from build123d import *

# Parameters (mm, degrees)
F0_R       = 5
F1_DEPTH   = 10
F2_R       = 7.5
F3_DEPTH   = 2
F4_C1_SIZE = 1
F4_C2_SIZE = 1
F4_C3_SIZE = 1
F4_C4_SIZE = 1
F4_C5_SIZE = 1
F4_C6_SIZE = 1
F4_C7_SIZE = 0.9999
F4_C8_SIZE = 1


# Not quite as in the source:
# - a fillet or chamfer is up to 0.001 mm smaller than in the source, because OpenCascade refuses the exact size


with BuildPart() as f1:
    # F0 (on Front) → F1 (new body)
    with BuildSketch(Plane.XZ):
        with BuildLine():
            ThreePointArc((3.1540486056, 9.4895720343), (1.5765683293, 9.7419684548), (0, 10))
            ThreePointArc((0, 10), (-10, 0), (0, -10))
            ThreePointArc((0, -10), (1.5765683293, -9.7419684548), (3.1540486056, -9.4895720343))
            ThreePointArc((3.1540486056, -9.4895720343), (8.1098855126, -5.8506202211), (10, 0))
            ThreePointArc((10, 0), (8.1098855126, 5.8506202211), (3.1540486056, 9.4895720343))
        make_face()
        Circle(F0_R, mode=Mode.SUBTRACT)
        with BuildLine():
            ThreePointArc((3.1540486056, 9.4895720343), (1.5975418081, 9.8715682731), (0, 10))
            ThreePointArc((0, 10), (1.5765683293, 9.7419684548), (3.1540486056, 9.4895720343))
        make_face()
        with BuildLine():
            ThreePointArc((3.1540486056, -9.4895720343), (1.5765683293, -9.7419684548), (0, -10))
            ThreePointArc((0, -10), (1.5975418081, -9.8715682731), (3.1540486056, -9.4895720343))
        make_face()
        with BuildLine():
            ThreePointArc((142.8459513944, 9.4895720343), (73, 4), (3.1540486056, 9.4895720343))
            ThreePointArc((3.1540486056, 9.4895720343), (8.1098855126, 5.8506202211), (10, 0))
            ThreePointArc((10, 0), (8.1098855126, -5.8506202211), (3.1540486056, -9.4895720343))
            ThreePointArc((3.1540486056, -9.4895720343), (73, -4), (142.8459513944, -9.4895720343))
            ThreePointArc((142.8459513944, -9.4895720343), (136, 0), (142.8459513944, 9.4895720343))
        make_face()
        with BuildLine():
            ThreePointArc((146, 10), (144.4234316707, 9.7419684548), (142.8459513944, 9.4895720343))
            ThreePointArc((142.8459513944, 9.4895720343), (136, 0), (142.8459513944, -9.4895720343))
            ThreePointArc((142.8459513944, -9.4895720343), (144.4234316707, -9.7419684548), (146, -10))
            ThreePointArc((146, -10), (153.0710678119, -7.0710678119), (156, 0))
            ThreePointArc((156, 0), (153.0710678119, 7.0710678119), (146, 10))
        make_face()
        with Locations((146, 0)):
            Circle(F0_R, mode=Mode.SUBTRACT)
        with BuildLine():
            ThreePointArc((146, 10), (144.4024581919, 9.8715682731), (142.8459513944, 9.4895720343))
            ThreePointArc((142.8459513944, 9.4895720343), (144.4234316707, 9.7419684548), (146, 10))
        make_face()
        with BuildLine():
            ThreePointArc((146, -10), (144.4234316707, -9.7419684548), (142.8459513944, -9.4895720343))
            ThreePointArc((142.8459513944, -9.4895720343), (144.4024581919, -9.8715682731), (146, -10))
        make_face()
    extrude(amount=F1_DEPTH)

    # F2 (on face) → F3 (cut)
    with BuildSketch(Plane.XZ.offset(10)):
        Circle(F2_R)
        with Locations((146, 0)):
            Circle(F2_R)
    extrude(amount=-F3_DEPTH, mode=Mode.SUBTRACT)

    # F4: chamfer of 1 on 8 edges, made by hand

    # F4_c1
    f4_c1_edges = [f1.edges().sort_by_distance(p)[0] for p in [
        (73, 0, -4),
    ]]
    chamfer(f4_c1_edges, length=F4_C1_SIZE)

    # F4_c2
    f4_c2_edges = [f1.edges().sort_by_distance(p)[0] for p in [
        (73, 0, 3.9999999999),
    ]]
    chamfer(f4_c2_edges, length=F4_C2_SIZE)

    # F4_c3
    f4_c3_edges = [f1.edges().sort_by_distance(p)[0] for p in [
        (-5, 0, 0),
    ]]
    chamfer(f4_c3_edges, length=F4_C3_SIZE)

    # F4_c4
    f4_c4_edges = [f1.edges().sort_by_distance(p)[0] for p in [
        (141, 0, 0),
    ]]
    chamfer(f4_c4_edges, length=F4_C4_SIZE)

    # F4_c5
    f4_c5_edges = [f1.edges().sort_by_distance(p)[0] for p in [
        (-5, -8, 0),
    ]]
    chamfer(f4_c5_edges, length=F4_C5_SIZE)

    # F4_c6
    f4_c6_edges = [f1.edges().sort_by_distance(p)[0] for p in [
        (141, -8, 0),
    ]]
    chamfer(f4_c6_edges, length=F4_C6_SIZE)

    # F4_c7 (size 1 in the source; OpenCascade refuses exactly that, so slightly less here)
    f4_c7_edges = [f1.edges().sort_by_distance(p)[0] for p in [
        (-10, 0, 0),
    ]]
    chamfer(f4_c7_edges, length=F4_C7_SIZE)

    # F4_c8
    f4_c8_edges = [f1.edges().sort_by_distance(p)[0] for p in [
        (156, 0, 0),
    ]]
    chamfer(f4_c8_edges, length=F4_C8_SIZE)


solid = f1.part
Work out the finished part from the listing and answer in its coordinate system (mm). A direction names the side the tool comes from. Round coordinates to 2 decimals unless told otherwise and drop trailing zeros. Write each loop counter-clockwise with the first axis right and the second up, starting at its lowest first coordinate (ties: lowest second). Pieces come first, ordered by that corner, then holes. Notation, with made-up numbers: M 64,9 L 77,9 A16 ccw 77,25 Z; hole C 16.25,56.5 d2. An arc over 180 degrees is marked long. Use a Markdown table: item, result.
1) Determine the mould class of faces 3 (the face through (74, -0.8, 3.8)), 4 (the face through (72, -10, 0)) for opening direction X: pulls with the +X half, pulls with the -X half, needs draft (parallel to the pull), parting line crosses it, or undercut.
Taken from the geometry:
| item | result |
|---|---|
| face 3 | undercut |
| face 4 | needs draft |
2) The part is cut by section A-A on y = -3.75. Give the vertices of the cut face in (x, z), plus the area to 3 significant figures.
Taken from the geometry:
| item | result |
|---|---|
| outline | M 3.15,-9.49 A447.08 cw 142.85,-9.49 A10 ccw long 142.85,9.49 A447.08 cw 3.15,9.49 A10 ccw long Z; hole C 0,0 d10; hole C 146,0 d10 |
| area | 1,910 mm2 |
3) Consider line 1 (X direction, y = -3.7, z = 0); line 2 (Z direction, x = 146, y = -2.3); line 3 (X direction, y = -7, z = 2.5). Determine where each line is inside the solid, lowest interval first. Write a range as [from, to].
Taken from the geometry:
| item | result |
|---|---|
| line 1 | x = [-10, -5], [5, 141], [151, 156] |
| line 2 | z = [-10, -5], [5, 10] |
| line 3 | x = [-9.68, -4.33], [4.33, 141.67], [150.33, 155.68] |
4) Which of the six approach directions +Z, -Z, +X, -X, +Y, -Y give full straight-line access (tool end or side, diameter ignored) to faces 1 (the face through (72, 0, 0)), 2 (the face through (-7.493, -9.014, 0.33))?
Taken from the geometry:
| item | result |
|---|---|
| face 1 | +Z, -Z, +X, -X, +Y |
| face 2 | -Y |
5) Flat-ended cylindrical pins translate along their axes: pin 1 (4 mm diameter, centred on x = 55.5, y = -2.5, fed in from +Z); pin 2 (3 mm diameter, centred on y = -1, z = -4, fed in from -X); pin 3 (6 mm diameter, centred on x = 146, z = 0, fed in from -Y); pin 4 (7.5 mm diameter, centred on x = 145, z = -1.5, fed in from -Y). Find the tip coordinate at first contact, or state that the pin passes through.
Taken from the geometry:
| item | result |
|---|---|
| pin 1 | stops at z = 4.43 |
| pin 2 | stops at x = -9.68 |
| pin 3 | passes through |
| pin 4 | stops at y = -7.55 |
